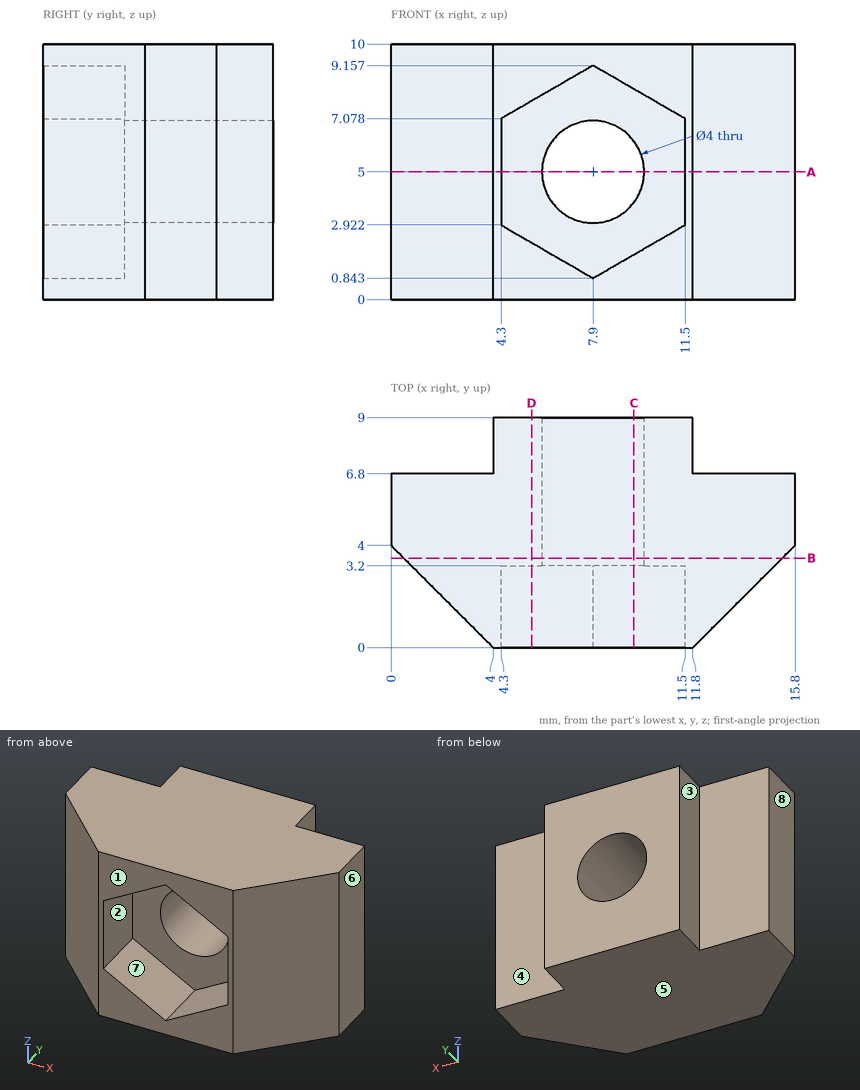
Could you check a few things on this drawing? It's one solid part, dimensions in mm from its lowest x, y, z. A direction names the side the tool comes from. Give positions to 0.01 mm unless a question says otherwise; leave off trailing zeros. Order: outer loops, then holes, each group sorted by start corner. A loop starts at its lowest first (then second) coordinate and runs counter-clockwise, first axis right, second up. Notation, with made-up numbers: M 21.5,-7.75 L 53.5,-7.75 A30 cw 53.5,27.25 Z; hole C 74.25,31.25 d10. An arc over 180 degrees is marked long. Use one line per item in the form item = value.
Item 1: Will these pins go through, and if not, where does the flat tip stop? pin 1 Ø1.2 at (x, z) = (2.5, 3) entering from +Y; pin 2 Ø2.5 at (y, z) = (1.5, 4.5) entering from +X; pin 3 Ø1 at (y, z) = (1.5, 3.5) entering from +X.
Values follow:
pin_1 = 6.8
pin_2 = 14.55
pin_3 = 13.8
Item 2: If we section it at C-C, the plane x = 9.5: Write out the boundary of the cut face in (y, z).
Values follow:
outline = M 0,0 L 9,0 L 9,3.8 L 3.2,3.8 L 3.2,1.77 L 0,1.77 Z; M 0,8.23 L 3.2,8.23 L 3.2,6.2 L 9,6.2 L 9,10 L 0,10 Z
Item 3: If I drill on line 1 along Z through (x, y) = (7.9, 6.5); line 2 along X through (y, z) = (7, 1.5); line 3 along X through (y, z) = (2, 2.75) (1 decimal), over which ranges is the centre line in solid material (lowest first)? Write a range as [from, to].
Values follow:
line_1 = [0, 3], [7, 10]
line_2 = [4, 11.8]
line_3 = [2, 4.6], [11.2, 13.8]
Item 4: If we section it at B-B, the plane y = 3.5: Write out the boundary of the cut face in (x, z), and give its area (3 significant figures).
Values follow:
outline = M 0.5,0 L 15.3,0 L 15.3,10 L 0.5,10 Z; hole C 7.9,5 d4
area = 135 mm^2
Item 5: Thinking about a two-plate mould opening in X: for the marked faces 6, 7 and 8, which applies, pulls with the +X half, pulls with the -X half, needs draft (parallel to the pull), parting line crosses it, or undercut?
Values follow:
face_6 = pulls with the +X half
face_7 = undercut
face_8 = pulls with the -X half
Item 6: If we section it at A-A, the plane z = 5: Write out the boundary of the cut face in (x, y).
Values follow:
outline = M 0,4 L 4,0 L 4.3,0 L 4.3,3.2 L 5.9,3.2 L 5.9,9 L 4,9 L 4,6.8 L 0,6.8 Z; M 9.9,3.2 L 11.5,3.2 L 11.5,0 L 11.8,0 L 15.8,4 L 15.8,6.8 L 11.8,6.8 L 11.8,9 L 9.9,9 Z
Item 7: If we section it at D-D, the plane x = 5.5: Write out the boundary of the cut face in (y, z).
Values follow:
outline = M 0,0 L 9,0 L 9,10 L 0,10 L 0,7.77 L 3.2,7.77 L 3.2,2.23 L 0,2.23 Z
Item 8: For the marked faces 1, 2, 3, 4 and 5, which set-ups out of +Z, -Z, +X, -X, +Y, -Y let a thin tool reach every point of the face, with its end or its side?
Values follow:
face_1 = +Z, -Z, +X, -X, -Y
face_2 = -Y
face_3 = +Z, -Z, -X, +Y
face_4 = +Z, -Z, +X, +Y
face_5 = -Z, +X, -X, +Y, -Y
